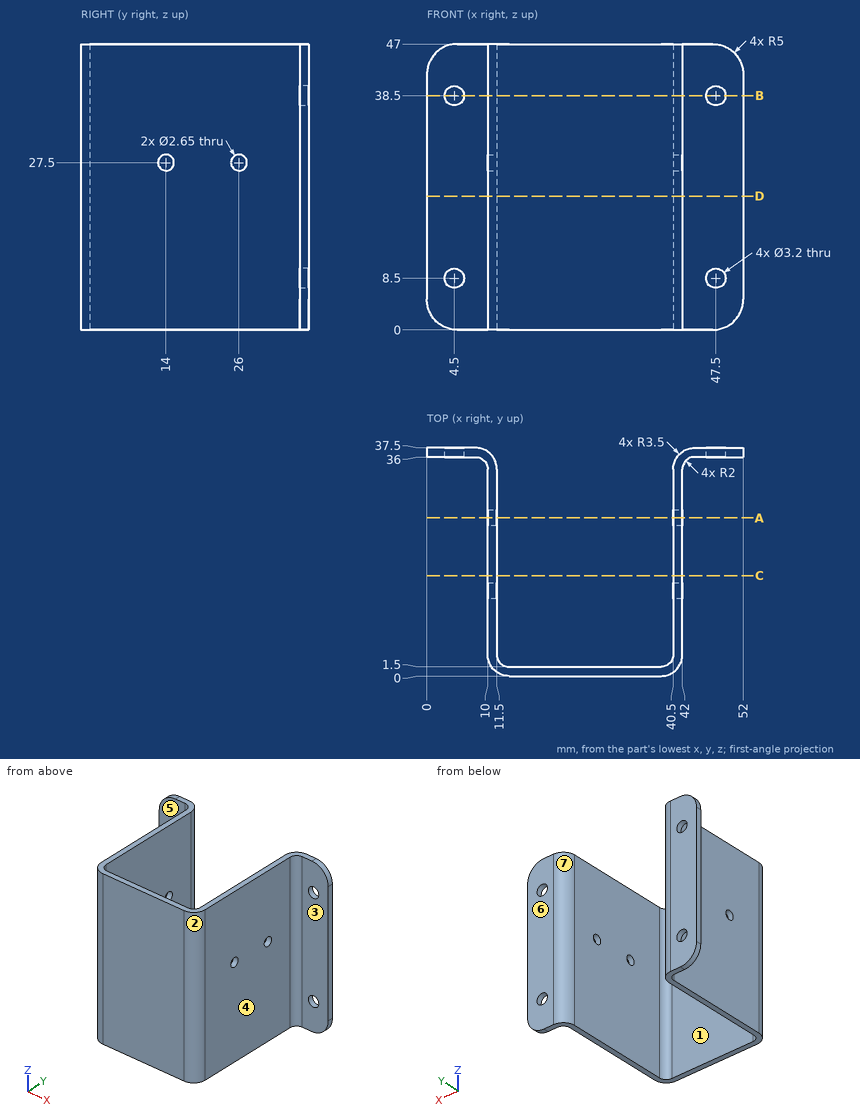
Input: dimensioned drawing with shaded views. Units: mm. Origin: part minimum x, y, z. A direction names the side the tool comes from. Coordinates: 2 decimals unless noted, no trailing zeros. Loops run counter-clockwise (first coordinate to the right, second up) from the corner with the lowest first, then second, coordinate; pieces in that order, holes last. Notation, with made-up numbers: (-26, 11.25) -> (12, 11.25) arc R23 ccw to (12, 27.25) -> close; hole circle Ø10 at (71.5, 21). An arc over 180 degrees is marked (long way). One line per item, written item: value. Start each with the question number.
Q1. Section query B-B, the plane z = 38.5. Return the cut outline in (x, y).
Q2. Line query: line 1 along X through (y, z) = (22, 30); line 2 along Y through (x, z) = (10.35, 27.5) (3 decimals); line 3 along X through (y, z) = (36.35, 8.5). Output: solid intervals per line, ascending.
Q3. Section query A-A, the plane y = 26. Return the cut outline in (x, z) (3 decimals).
Q4. Set-up query: the marked faces 4, 5, 6 and 7. Return all of +Z, -Z, +X, -X, +Y, -Y with unobstructed straight access to the full face (end or side cutting, diameter ignored); none if empty.
Q5. Mould query, pull axis X, two halves, no side actions, for the marked faces 1, 2 and 3. Classes: pulls with the +X half, pulls with the -X half, needs draft (parallel to the pull), parting line crosses it, or undercut.
Q6. Section query D-D, the plane z = 22. Return the cut outline in (x, y).
Q7. Contact query for flat-ended pins moving along their axis: P1, Ø12, axis at y = 6.5, z = 9.5, coming from the +X side; P2, Ø4, axis at x = 47.5, z = 38.5, coming from the -Y side; P3, Ø10, axis at x = 19, z = 26, coming from the -Y side; P4, Ø9, axis at x = 48, z = 31.5, coming from the -Y side. Output: stop coordinate, or through.
Q8. Section query C-C, the plane y = 16.5. Return the cut outline in (x, z), and give its area (3 significant figures).
Results:
1. outline: (0, 36) -> (2.9, 36) -> (2.9, 37.5) -> (0, 37.5) -> close; (6.1, 36) -> (8, 36) arc R2 cw to (10, 34) -> (10, 3.5) arc R3.5 ccw to (13.5, 0) -> (38.5, 0) arc R3.5 ccw to (42, 3.5) -> (42, 34) arc R2 cw to (44, 36) -> (45.9, 36) -> (45.9, 37.5) -> (44, 37.5) arc R3.5 ccw to (40.5, 34) -> (40.5, 3.5) arc R2 cw to (38.5, 1.5) -> (13.5, 1.5) arc R2 cw to (11.5, 3.5) -> (11.5, 34) arc R3.5 ccw to (8, 37.5) -> (6.1, 37.5) -> close; (49.1, 36) -> (52, 36) -> (52, 37.5) -> (49.1, 37.5) -> close
2. line 1: 10 to 11.5, 40.5 to 42
2. line 2: 1.974 to 12.675, 15.325 to 24.675, 27.325 to 36.594
2. line 3: 0 to 2.9, 6.1 to 10.59, 41.41 to 45.9, 49.1 to 52
3. outline: (10, 0) -> (11.5, 0) -> (11.5, 26.175) -> (10, 26.175) -> close; (10, 28.825) -> (11.5, 28.825) -> (11.5, 47) -> (10, 47) -> close; (40.5, 0) -> (42, 0) -> (42, 26.175) -> (40.5, 26.175) -> close; (40.5, 28.825) -> (42, 28.825) -> (42, 47) -> (40.5, 47) -> close
4. face 4: +Z, -Z, +X, -Y
4. face 5: +Z, -Z, -X, -Y
4. face 6: +Z, -Z, +X, -X, +Y
4. face 7: +Z, -Z, +Y
5. face 1: undercut
5. face 2: pulls with the +X half
5. face 3: needs draft
6. outline: (0, 36) -> (8, 36) arc R2 cw to (10, 34) -> (10, 3.5) arc R3.5 ccw to (13.5, 0) -> (38.5, 0) arc R3.5 ccw to (42, 3.5) -> (42, 34) arc R2 cw to (44, 36) -> (52, 36) -> (52, 37.5) -> (44, 37.5) arc R3.5 ccw to (40.5, 34) -> (40.5, 3.5) arc R2 cw to (38.5, 1.5) -> (13.5, 1.5) arc R2 cw to (11.5, 3.5) -> (11.5, 34) arc R3.5 ccw to (8, 37.5) -> (0, 37.5) -> close
7. P1: x = 42
7. P2: y = 36
7. P3: y = 0
7. P4: y = 35.94
8. outline: (10, 0) -> (11.5, 0) -> (11.5, 47) -> (10, 47) -> close; (40.5, 0) -> (42, 0) -> (42, 47) -> (40.5, 47) -> close
8. area: 141 mm^2
